The model under review builds one solid part; all positions refer to its coordinate system, in mm. Face numbers are marked on the shaded views. Coordinates: 2 decimals unless noted, no trailing zeros. Loops run counter-clockwise (first coordinate to the right, second up) from the corner with the lowest first, then second, coordinate; pieces in that order, holes last. Notation, with made-up numbers: (42, 63.5) - (48, 63.5) arc R17 ccw to (48, 94.5) - close; hole circle Ø6 at (-11, 42). An arc over 180 degrees is marked (long way). One line per item, written item: value. Start each with the question number.
1. We need section A-A, the plane x = 0. Give the boundary of the cut face in (y, z).
2. Mouldability with a two-part tool opening along X and no side actions: class the marked faces 1, 2, 3 and 4 as +X half, -X half, draft (parallel to the pull), parting line (faces both ways), or undercut.
3. Insertion check: P1, Ø3, axis at x = 14.5, z = 25, coming from the -Y side; P2, Ø4, axis at x = -13, z = 6.5, coming from the -Y side; P3, Ø5.5, axis at x = -14.5, z = 5, coming from the -Y side; P4, Ø5, axis at x = 10, y = 6.5, coming from the -Z side. Each pin has a flat end and moves straight along its axis. Give the tip position at first contact, or say it passes through.
4. We need section D-D, the plane x = -10. Give the boundary of the cut face in (y, z), then the cut area to 3 significant figures.
5. We need section B-B, the plane z = 16.5. Give the boundary of the cut face in (x, y).
6. We need section C-C, the plane z = 8. Give the boundary of the cut face in (x, y), then the cut area to 3 significant figures.
7. To check wall thickness, follow line 1 (Y direction, x = 0, z = 29); line 2 (Y direction, x = 0, z = 6.5); line 3 (Z direction, x = 11.8, y = 6.5). State the ranges of each line that lie inside material, in increasing order.
from build123d import *

# Parameters (mm, degrees)
EXTRUDE_1_DEPTH             = 50
SKETCH_2_OUTSIDE_W          = 51.398
SKETCH_2_OUTSIDE_H          = 41.698
SKETCH_2_OUTSIDE_R          = 7
CUT_EXTRUDE_3_DEPTH         = 10
SKETCH_5_R                  = 11
CUT_EXTRUDE_5_DEPTH         = 27
HOLE_WIZARD_M4_1_AT_2_COUNT = 2
HOLE_WIZARD_M4_1_AT_2_PITCH = 20
HOLE_WIZARD_M4_1_AT_3_COUNT = 2
HOLE_WIZARD_M4_1_AT_3_PITCH = 40
CUT_EXTRUDE_1_DEPTH         = 34
HOLE_WIZARD_3_0_3_1_REACH   = 65.031
HOLE_WIZARD_3_0_3_1_BORE_R  = 1.5
SKETCH_65_R                 = 2
CUT_EXTRUDE_2_DEPTH         = 5


with BuildPart() as part:
    # 草图1 → 拉伸1 (new body)
    with BuildSketch(Plane.XY):
        Polygon((-18, 13), (-18, -3), (-7, -13.3), (7, -13.3), (18, -3), (18, 13), align=None)
    extrude(amount=EXTRUDE_1_DEPTH)

    # 草图2 outside → 拉伸3 (cut)
    # profile 1 of 2: a face of its own
    with BuildSketch(Plane.XY.offset(50)):
        with Locations((0, -0.15)):
            Rectangle(SKETCH_2_OUTSIDE_W, SKETCH_2_OUTSIDE_H)
        Polygon((18, -3), (18, 13), (-18, 13), (-18, -3), (-7, -13.3), (7, -13.3), align=None, mode=Mode.SUBTRACT)
    # profile 2 of 2: a face of its own
    with BuildSketch(Plane.XY.offset(50)):
        Circle(SKETCH_2_OUTSIDE_R)
    extrude(amount=-CUT_EXTRUDE_3_DEPTH, mode=Mode.SUBTRACT)

    # 草图5 → 拉伸5 (cut)
    with BuildSketch(Plane.XY.offset(40)):
        Circle(SKETCH_5_R)
    extrude(amount=-CUT_EXTRUDE_5_DEPTH, mode=Mode.SUBTRACT)

    # 草图57 → M24 螺纹孔1 (revolve, cut)
    with BuildSketch(Plane(origin=(0, 0, 13), x_dir=(0, -1, 0), z_dir=(1, 0, 0))):
        Polygon((0, 0), (0, 19.909897119), (11.5, 13), (11.5, 0), align=None)
    revolve(axis=Axis((0, 0, 19.35), (0, 0, -1)), mode=Mode.SUBTRACT)

    # 草图58 → M4 螺纹孔1 (revolve, cut)
    with BuildSketch(Plane(origin=(-14.5, 13, 5), x_dir=(0, 0, 1), z_dir=(1, 0, 0))):
        Polygon((0, 0), (0, 12.491420021), (1.65, 11.5), (1.65, 0), align=None)
    hole_wizard_m4_1 = revolve(axis=Axis((-14.5, 19.35, 5), (0, -1, 0)), mode=Mode.SUBTRACT)

    # M4 螺纹孔1 at 2: M4 螺纹孔1 ×2
    with Locations(*[(0, 0, i * HOLE_WIZARD_M4_1_AT_2_PITCH) for i in range(1, HOLE_WIZARD_M4_1_AT_2_COUNT)]):
        add(hole_wizard_m4_1, mode=Mode.SUBTRACT)

    # M4 螺纹孔1 at 3: M4 螺纹孔1 ×2
    with Locations(*[(0, 0, i * HOLE_WIZARD_M4_1_AT_3_PITCH) for i in range(1, HOLE_WIZARD_M4_1_AT_3_COUNT)]):
        add(hole_wizard_m4_1, mode=Mode.SUBTRACT)

    # 镜向1: M4 螺纹孔1 across plane
    add(hole_wizard_m4_1.mirror(Plane(origin=(0, 0, 0), x_dir=(0, 0, 1), z_dir=(1, 0, 0))), mode=Mode.SUBTRACT)

    # 镜向1 copy 1 sketch → 镜向1 copy 1 (revolve, cut)
    with BuildSketch(Plane(origin=(14.5, 13, 25), x_dir=(0, 0, 1), z_dir=(-1, 0, 0))):
        Polygon((0, 0), (0, -12.491420021), (1.65, -11.5), (1.65, 0), align=None)
    revolve(axis=Axis((14.5, 19.35, 25), (0, 1, 0)), mode=Mode.SUBTRACT)

    # 镜向1 copy 2 sketch → 镜向1 copy 2 (revolve, cut)
    with BuildSketch(Plane(origin=(14.5, 13, 45), x_dir=(0, 0, 1), z_dir=(-1, 0, 0))):
        Polygon((0, 0), (0, -12.491420021), (1.65, -11.5), (1.65, 0), align=None)
    revolve(axis=Axis((14.5, 19.35, 45), (0, 1, 0)), mode=Mode.SUBTRACT)

    # 草图61 → 切除-拉伸1 (cut)
    with BuildSketch(Plane(origin=(0, 0, 0), x_dir=(-1, 0, 0), z_dir=(0, 0, -1))):
        with BuildLine():
            Line((-9.337993294, 8.980082474), (1.147152873, 1.638304089))
            ThreePointArc((1.147152873, 1.638304089), (1.638304089, -1.147152873), (-1.147152873, -1.638304089))
            Line((-1.147152873, -1.638304089), (-11.63229904, 5.703474297))
            ThreePointArc((-11.63229904, 5.703474297), (-12.123450255, 8.488931258), (-9.337993294, 8.980082474))
        make_face()
    extrude(amount=-CUT_EXTRUDE_1_DEPTH, mode=Mode.SUBTRACT)

    # Ø3.0 (3) 直径孔1 bore → Ø3.0 (3) 直径孔1 (cut, up to next)
    with BuildSketch(Plane(origin=(18, 0, 0), x_dir=(0, 0, -1), z_dir=(1, 0, 0)), mode=Mode.PRIVATE) as hole_wizard_3_0_3_1_sk1:
        with Locations((-32, 6.5)):
            Circle(HOLE_WIZARD_3_0_3_1_BORE_R)
    hole_wizard_3_0_3_1_tool1 = extrude(hole_wizard_3_0_3_1_sk1.sketch, amount=-HOLE_WIZARD_3_0_3_1_REACH, mode=Mode.PRIVATE) & part.part
    add(hole_wizard_3_0_3_1_tool1.solids().sort_by_distance((18, 6.5, 32))[0], mode=Mode.SUBTRACT)

    # 草图65 → 切除-拉伸2 (cut)
    with BuildSketch(Plane(origin=(18, 0, 0), x_dir=(0, 0, -1), z_dir=(1, 0, 0))):
        with Locations((-32, 6.5)):
            Circle(SKETCH_65_R)
    extrude(amount=-CUT_EXTRUDE_2_DEPTH, mode=Mode.SUBTRACT)


solid = part.part
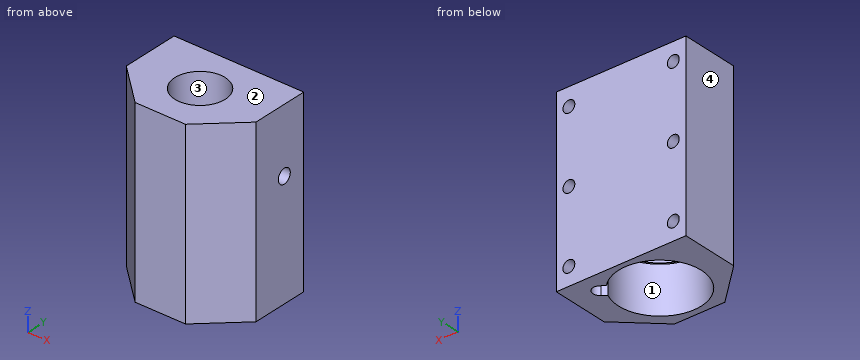
Findings below:
1. outline: (-13.3, 0) - (-11.5, 0) - (-11.5, 13) - (-11, 13) - (-11, 40) - (-7, 40) - (-7, 50) - (-13.3, 50) - close; (7, 40) - (11, 40) - (11, 13) - (11.5, 13) - (11.5, 0) - (13, 0) - (13, 50) - (7, 50) - close
2. face 1: undercut
2. face 2: draft
2. face 3: undercut
2. face 4: -X half
3. P1: y = -7.68
3. P2: y = -9.55
3. P3: y = -8.85
3. P4: z = 0
4. outline: (-10.49, 0) - (-5.68, 0) - (-5.68, 13) - (-4.58, 13) - (-4.58, 40) - (4.58, 40) - (4.58, 13) - (5.68, 13) - (5.68, 0) - (13, 0) - (13, 50) - (-10.49, 50) - close
4. area: 779 mm2
5. outline: (-18, -3) - (-7, -13.3) - (7, -13.3) - (18, -3) - (18, 13) - (-18, 13) - close; hole (7.71, 7.84) arc R11 ccw (long way) to (10.01, 4.57) - (11.63, 5.7) arc R2 ccw to (9.34, 8.98) - close
6. outline: (-18, -3) - (-7, -13.3) - (7, -13.3) - (18, -3) - (18, 13) - (-18, 13) - close; hole (8.13, 8.13) arc R11.5 ccw (long way) to (10.42, 4.86) - (11.63, 5.7) arc R2 ccw to (9.34, 8.98) - close
6. area: 406 mm2
7. line 1: -13.3 to -11, 11 to 13
7. line 2: -13.3 to -11.5, 11.5 to 13
7. line 3: 34 to 50
